Check sheet for the modelled part. Datum: model origin and axes. Units: mm. A direction names the side the tool comes from. Give positions to 0.01 mm unless a question says otherwise; leave off trailing zeros. Order: outer loops, then holes, each group sorted by start corner. A loop starts at its lowest first (then second) coordinate and runs counter-clockwise, first axis right, second up.
```python
from build123d import *

# Parameters (mm, degrees)
SKETCH1_R           = 8.5
BOSS_EXTRUDE1_DEPTH = 2
CUT_EXTRUDE1_START  = -0.5
CUT_EXTRUDE1_DEPTH  = 0.5
BOSS_EXTRUDE2_START = -37
BOSS_EXTRUDE2_DEPTH = 37
BOSS_EXTRUDE4_DEPTH = 8
BOSS_EXTRUDE5_DEPTH = 1.236037686
SKETCH11_R          = 5
BOSS_EXTRUDE6_DEPTH = 34.7
SKETCH12_R          = 2.8
CUT_EXTRUDE2_DEPTH  = 6
DRAFT1_ANGLE        = -1
SKETCH16_R          = 2.8
CUT_EXTRUDE3_DEPTH  = 29
SKETCH17_R          = 1.35
CUT_EXTRUDE4_DEPTH  = 29


# Read off the part's stored shape, not the designer's step: Mirror5
with BuildPart() as part:
    # Sketch1 → Boss-Extrude1 (new body)
    with BuildSketch(Plane.XY):
        with BuildLine():
            Line((-70, 0), (-70, -38))
            Line((-70, -38), (-66, -38))
            ThreePointArc((-66, -38), (0, -17.5), (66, -38))
            Line((66, -38), (70, -38))
            Line((70, -38), (70, 0))
            ThreePointArc((70, 0), (0, 70), (-70, 0))
        make_face()
        with Locations((0, 43.5)):
            Circle(SKETCH1_R, mode=Mode.SUBTRACT)
    extrude(amount=BOSS_EXTRUDE1_DEPTH)

    # Sketch2 → Cut-Extrude1 (cut)
    with BuildSketch(Plane.XY.offset(2).offset(CUT_EXTRUDE1_START)):
        with BuildLine():
            Line((-70, 0), (-70, -38))
            Line((-70, -38), (-66, -38))
            ThreePointArc((-66, -38), (0, -17.5), (66, -38))
            Line((66, -38), (70, -38))
            Line((70, -38), (70, 0))
            ThreePointArc((70, 0), (0, 70), (-70, 0))
        make_face()
        with BuildLine():
            Line((-69.5, 0), (-69.5, -37.5))
            Line((-69.5, -37.5), (-66.155120739, -37.5))
            ThreePointArc((-66.155120739, -37.5), (0, -17), (66.155120739, -37.5))
            Line((66.155120739, -37.5), (69.5, -37.5))
            Line((69.5, -37.5), (69.5, 0))
            ThreePointArc((69.5, 0), (0, 69.5), (-69.5, 0))
        make_face(mode=Mode.SUBTRACT)
    extrude(amount=CUT_EXTRUDE1_DEPTH, mode=Mode.SUBTRACT)

    # Sketch5 → Boss-Extrude2 (add)
    with BuildSketch(Plane.XY.offset(BOSS_EXTRUDE2_START)):
        with BuildLine():
            Line((66.849829887, -36.763962314), (70, -36.763962314))
            Line((70, -36.763962314), (70, -38))
            Line((70, -38), (66, -38))
            ThreePointArc((66, -38), (0, -17.5), (-66, -38))
            Line((-66, -38), (-70, -38))
            Line((-70, -38), (-70, -36.763962314))
            Line((-70, -36.763962314), (-66.849829887, -36.763962314))
            ThreePointArc((-66.849829887, -36.763962314), (0, -16), (66.849829887, -36.763962314))
        make_face()
    boss_extrude2 = extrude(amount=BOSS_EXTRUDE2_DEPTH)

    # Sketch9 → Boss-Extrude4 (add)
    with BuildSketch(Plane(origin=(0, -38, 0), x_dir=(1, 0, 0), z_dir=(0, 1, 0))):
        with BuildLine():
            ThreePointArc((-78.8, -0.5), (-93.295689014, 5.504310986), (-99.3, 20))
            Line((-99.3, 20), (-99.3, 37))
            Line((-99.3, 37), (-98.8, 37))
            Line((-98.8, 37), (-98.8, 20))
            ThreePointArc((-98.8, 20), (-92.942135624, 5.857864376), (-78.8, 0))
            Line((-78.8, 0), (-70, 0))
            Line((-70, 0), (-70, -0.5))
            Line((-70, -0.5), (-78.8, -0.5))
        make_face()
    boss_extrude4 = extrude(amount=BOSS_EXTRUDE4_DEPTH)

    # Sketch10 → Boss-Extrude5 (add)
    with BuildSketch(Plane(origin=(0, -38, 0), x_dir=(1, 0, 0), z_dir=(0, 1, 0))):
        with BuildLine():
            Line((-70, 0), (-78.8, 0))
            ThreePointArc((-78.8, 0), (-92.942135624, 5.857864376), (-98.8, 20))
            Line((-98.8, 20), (-98.8, 37))
            Line((-98.8, 37), (-70, 37))
            Line((-70, 37), (-70, 0))
        make_face()
    boss_extrude5 = extrude(amount=BOSS_EXTRUDE5_DEPTH)

    # Sketch11 → Boss-Extrude6 (add)
    with BuildSketch(Plane(origin=(0, -36.763962314, 0), x_dir=(1, 0, 0), z_dir=(0, 1, 0))):
        with Locations(Location((-83.3, 8.1, 0), (0, 0, 270))):
            Circle(SKETCH11_R)
    boss_extrude6 = extrude(amount=BOSS_EXTRUDE6_DEPTH)

    # Sketch12 → Cut-Extrude2 (cut)
    with BuildSketch(Plane(origin=(0, -2.063962314, 0), x_dir=(1, 0, 0), z_dir=(0, 1, 0))):
        with Locations(Location((-83.3, 8.1, 0), (0, 0, 270))):
            Circle(SKETCH12_R)
    cut_extrude2 = extrude(amount=-CUT_EXTRUDE2_DEPTH, mode=Mode.SUBTRACT)

    # Draft1
    draft1_faces = [part.faces().sort_by_distance(p)[0] for p in [
        (-83.3, -5.063962314, -10.9),
    ]]
    draft(draft1_faces, Plane(origin=(-83.3, -8.063962314, -8.1), x_dir=(0, 0, 1), z_dir=(0, 1, 0)), DRAFT1_ANGLE)

    # Sketch14 → Cut-Revolve2 (revolve, cut)
    with BuildSketch(Plane.XY.offset(-8.1), mode=Mode.PRIVATE) as cut_revolve2_sk:
        Polygon((-85.99526961, -2.063962314), (-86.1, -8.063962314), (-88.3, -2.063962314), align=None)
    cut_revolve2 = revolve(cut_revolve2_sk.sketch.rotate(Axis((-83.3, -8.063962314, -8.1), (0, 1, 0)), 270), axis=Axis((-83.3, -8.063962314, -8.1), (0, 1, 0)), mode=Mode.SUBTRACT)

    # Mirror3: Boss-Extrude2, Boss-Extrude4, Boss-Extrude5, Boss-Extrude6, Cut-Extrude2, Cut-Revolve2 across plane
    add(boss_extrude2.mirror(Plane(origin=(0, 0, 0), x_dir=(0, 0, 1), z_dir=(1, 0, 0))))
    add(boss_extrude4.mirror(Plane(origin=(0, 0, 0), x_dir=(0, 0, 1), z_dir=(1, 0, 0))))
    add(boss_extrude5.mirror(Plane(origin=(0, 0, 0), x_dir=(0, 0, 1), z_dir=(1, 0, 0))))
    add(boss_extrude6.mirror(Plane(origin=(0, 0, 0), x_dir=(0, 0, 1), z_dir=(1, 0, 0))))
    add(cut_extrude2.mirror(Plane(origin=(0, 0, 0), x_dir=(0, 0, 1), z_dir=(1, 0, 0))), mode=Mode.SUBTRACT)
    add(cut_revolve2.mirror(Plane(origin=(0, 0, 0), x_dir=(0, 0, 1), z_dir=(1, 0, 0))), mode=Mode.SUBTRACT)

    # Mirror5: part across plane


with BuildPart() as part_1:
    add(part.part)
    add(part.part.mirror(Plane(origin=(0, -133.993902439, -37), x_dir=(1, 0, 0), z_dir=(0, 0, 1))))

    # Sketch16 → Cut-Extrude3 (cut)
    with BuildSketch(Plane.XZ.offset(38)):
        with Locations(Location((-83.3, -65.9, 0), (0, 0, 270))):
            Circle(SKETCH16_R)
        with Locations(Location((83.3, -65.9, 0), (0, 0, 270))):
            Circle(SKETCH16_R)
        with Locations(Location((83.3, -8.1, 0), (0, 0, 270))):
            Circle(SKETCH16_R)
        with Locations(Location((-83.3, -8.1, 0), (0, 0, 270))):
            Circle(SKETCH16_R)
    extrude(amount=-CUT_EXTRUDE3_DEPTH, mode=Mode.SUBTRACT)

    # Sketch17 → Cut-Extrude4 (cut)
    with BuildSketch(Plane(origin=(0, -8.063962314, 0), x_dir=(1, 0, 0), z_dir=(0, 1, 0))):
        with Locations(Location((-83.3, 65.9, 0), (0, 0, 270))):
            Circle(SKETCH17_R)
        with Locations(Location((-83.3, 8.1, 0), (0, 0, 270))):
            Circle(SKETCH17_R)
        with Locations(Location((83.3, 65.9, 0), (0, 0, 270))):
            Circle(SKETCH17_R)
        with Locations(Location((83.3, 8.1, 0), (0, 0, 270))):
            Circle(SKETCH17_R)
    extrude(amount=-CUT_EXTRUDE4_DEPTH, mode=Mode.SUBTRACT)


solid = part_1.part
```
(1) Cross-section at C-C on z = -25. Enter the section's corners in (x, y), then the cut area to 3 significant figures.
Response values:
outline: (-99.3, -38) - (-66, -38) arc R116.49 cw to (66, -38) - (99.3, -38) - (99.3, -30) - (98.8, -30) - (98.8, -36.76) - (66.85, -36.76) arc R117.99 ccw to (-66.85, -36.76) - (-98.8, -36.76) - (-98.8, -30) - (-99.3, -30) - close
area: 300 mm2
(2) Cross-section at A-A on y = -5.5. Count the separate pieces of the cut face and the enclosed holes in it, then the cut area to 3 significant figures.
Response values:
separate pieces: 6
enclosed holes: 4
area: 697 mm2
(3) Material ranges on L1, parallel to X at y = -8, z = -8; L2, parallel to Z at x = 83, y = -8; L3, parallel to X at y = -8.35, z = -8.1, recorded low to high.
Response values:
L1: x = -88.3 to -86.12, -80.48 to -78.3, 78.3 to 80.48, 86.12 to 88.3
L2: z = -70.89 to -68.71, -63.09 to -60.91, -13.09 to -10.91, -5.29 to -3.11
L3: x = -88.3 to -84.65, -81.95 to -78.3, 78.3 to 81.95, 84.65 to 88.3
(4) Cross-section at B-B on x = 0. Enter the section's corners in (y, z), then the cut area to 3 significant figures.
Response values:
outline: (-17.5, -75.5) - (-17, -75.5) - (-17, -76) - (35, -76) - (35, -74) - (-16, -74) - (-16, 0) - (35, 0) - (35, 2) - (-17, 2) - (-17, 1.5) - (-17.5, 1.5) - close; (52, -76) - (69.5, -76) - (69.5, -75.5) - (70, -75.5) - (70, -74) - (52, -74) - close; (52, 0) - (70, 0) - (70, 1.5) - (69.5, 1.5) - (69.5, 2) - (52, 2) - close
area: 392 mm2
(5) Release check for a two-part mould opening along Z. For faces 4 (the face through (74, -34, 0.5)), 5 (the face through (1.539, 69.983, -74.74)), 6 (the face through (86.3, -19.7, -61.9)) record: released by +Z, released by -Z, zero draft, split by the parting line, or undercut.
Response values:
face 4: released by +Z
face 5: zero draft
face 6: undercut
(6) Cross-section at D-D on y = 30. Enter the section's corners in (x, z), then the cut area to 3 significant figures.
Response values:
outline: (-63.25, -75.5) - (-62.69, -75.5) - (-62.69, -76) - (62.69, -76) - (62.69, -75.5) - (63.25, -75.5) - (63.25, -74) - (-63.25, -74) - close; (-63.25, 0) - (63.25, 0) - (63.25, 1.5) - (62.69, 1.5) - (62.69, 2) - (-62.69, 2) - (-62.69, 1.5) - (-63.25, 1.5) - close
area: 505 mm2
(7) Gauge pin test, flat ends, axial feed: pin 1 Ø2 at (x, z) = (-51, -7.5) entering from -Y; pin 2 Ø3.5 at (x, z) = (-83.3, -65.9) entering from +Y; pin 3 Ø1.2 at (y, z) = (-11.5, -75) entering from +X. Record the tip position at first contact, or that the pin passes through.
Response values:
pin 1: stops at y = -29.75
pin 2: stops at y = -8.06
pin 3: stops at x = 70
(8) Set-up check for faces 1 (the face through (1.528, 69.483, -75.746)), 2 (the face through (-85, -8.064, -9)), 3 (the face through (-74, -34, 0.5)): record each of +Z, -Z, +X, -X, +Y, -Y from which the full face is reachable in a straight line by a thin tool's end or side.
Response values:
face 1: -Z, +Y
face 2: +Y
face 3: +Z, -X, +Y, -Y
